Design review of the part built by this model. Coordinates are the model's own, in mm. Face numbers are marked on the shaded views. Give positions to 0.01 mm unless a question says otherwise; leave off trailing zeros. Loops run counter-clockwise (first coordinate to the right, second up) from the corner with the lowest first, then second, coordinate; pieces in that order, holes last. Notation, with made-up numbers: (10.5, 89.5) - (59.5, 89.5) arc R29 cw to (59.5, 126.5) - close; hole circle Ø9 at (31.25, -4.75). An arc over 180 degrees is marked (long way). Put each result on its own line as item: value. Start each with the question number.
```python
from build123d import *

# Parameters (mm, degrees)
F0_W     = 25.4
F0_H     = 25.4
F0_R     = 6.35
F0_W_2   = 12.7
F0_H_2   = 12.7
F0_R_2   = 3.175
F1_DEPTH = 30.48
F2_W     = 27.94
F2_H     = 12.7
F3_DEPTH = 12.7


with BuildPart() as f1:
    # F0 (on Front) → F1 (new body)
    with BuildSketch(Plane.XZ):
        with Locations((0, 38.1)):
            Rectangle(F0_W, F0_H)
        with Locations((0, 38.1)):
            Circle(F0_R, mode=Mode.SUBTRACT)
        Polygon((12.7, 25.4), (-12.7, 25.4), (-12.7, -50.8), (12.7, -50.8), (12.7, -12.7), (12.7, 0), align=None)
        with Locations((19.05, -6.35)):
            Rectangle(F0_W_2, F0_H_2)
        with Locations((19.05, -6.35)):
            Circle(F0_R_2, mode=Mode.SUBTRACT)
    extrude(amount=F1_DEPTH)

    # F2 (on face) → F3 (cut)
    with BuildSketch(Plane.YZ.offset(25.4)):
        with Locations((-15.24, -6.35)):
            Rectangle(F2_W, F2_H)
    extrude(amount=-F3_DEPTH, mode=Mode.SUBTRACT)


solid = f1.part
```
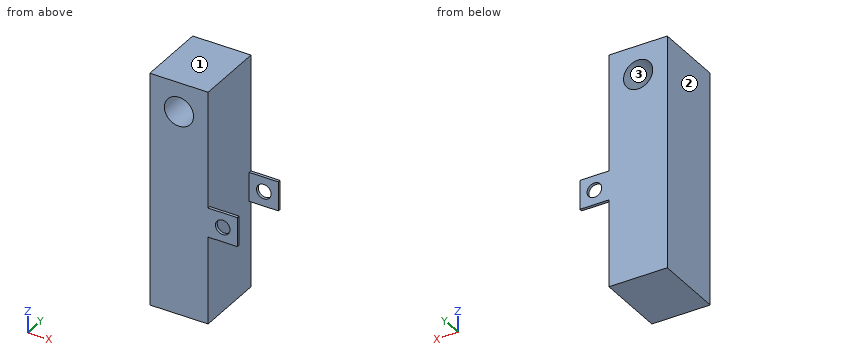
Item 1: Consider section D-D (x = 20.5). State the section outline as (y, z) points.
Item 2: Mouldability with a two-part tool opening along X and no side actions: class the marked faces 1, 2 and 3 as pulls with the +X half, pulls with the -X half, needs draft (parallel to the pull), parting line crosses it, or undercut.
Item 3: Consider section B-B (z = 38.1). State the section outline as (x, y) points.
Item 4: Consider section A-A (x = 0). State the section outline as (y, z) points, plus the area to 3 significant figures.
Item 5: For L1, parallel to Z at x = 0, y = -24; L2, parallel to X at y = -0.75, z = -6.35 (3 decimals); L3, parallel to Z at x = 19, y = -30, list the stretches that pass through material, from the lowest coordinate up. Write a range as from..to.
Item 6: For P1, Ø20.5, axis at x = 0, z = 38.1, coming from the +Y side; P2, Ø12, axis at x = 19, y = -10.5, coming from the +Z side; P3, Ø0.6, axis at x = 21.5, y = -30, coming from the -Z side; P4, Ø4, axis at y = -14, z = -19, coming from the +X side, all flat-tipped, find the tip position at first contact; note any pin that passes through.
Item 7: Consider section C-C (z = -6.35). State the section outline as (x, y) points (3 decimals).
Geometry says:
1. outline: (-30.48, -12.7) - (-29.21, -12.7) - (-29.21, -9.17) - (-30.48, -9.17) - close; (-30.48, -3.53) - (-29.21, -3.53) - (-29.21, 0) - (-30.48, 0) - close; (-1.27, -12.7) - (0, -12.7) - (0, -9.17) - (-1.27, -9.17) - close; (-1.27, -3.53) - (0, -3.53) - (0, 0) - (-1.27, 0) - close
2. face 1: needs draft
2. face 2: pulls with the -X half
2. face 3: undercut
3. outline: (-12.7, -30.48) - (-6.35, -30.48) - (-6.35, 0) - (-12.7, 0) - close; (6.35, -30.48) - (12.7, -30.48) - (12.7, 0) - (6.35, 0) - close
4. outline: (-30.48, -50.8) - (0, -50.8) - (0, 31.75) - (-30.48, 31.75) - close; (-30.48, 44.45) - (0, 44.45) - (0, 50.8) - (-30.48, 50.8) - close
4. area: 2,710 mm2
5. L1: z = -50.8..31.75, 44.45..50.8
5. L2: x = -12.7..15.875, 22.225..25.4
5. L3: z = -12.7..-9.52, -3.18..0
6. P1: stops at y = 0
6. P2: passes through
6. P3: stops at z = -12.7
6. P4: stops at x = 12.7
7. outline: (-12.7, -30.48) - (15.875, -30.48) - (15.875, -29.21) - (12.7, -29.21) - (12.7, -1.27) - (15.875, -1.27) - (15.875, 0) - (-12.7, 0) - close; (22.225, -30.48) - (25.4, -30.48) - (25.4, -29.21) - (22.225, -29.21) - close; (22.225, -1.27) - (25.4, -1.27) - (25.4, 0) - (22.225, 0) - close
